Input: dimensioned drawing with shaded views. Units: mm. Origin: part minimum x, y, z. A direction names the side the tool comes from. Round coordinates to 2 decimals unless told otherwise and drop trailing zeros. Write each loop counter-clockwise with the first axis right and the second up, starting at its lowest first coordinate (ties: lowest second). Pieces come first, ordered by that corner, then holes. Notation, with made-up numbers: (5, 71.5) - (45, 71.5) arc R29 ccw to (45, 103.5) - close; hole circle Ø2 at (85.5, -10.75). An arc over 180 degrees is marked (long way). Use one line per item in the form item = value.
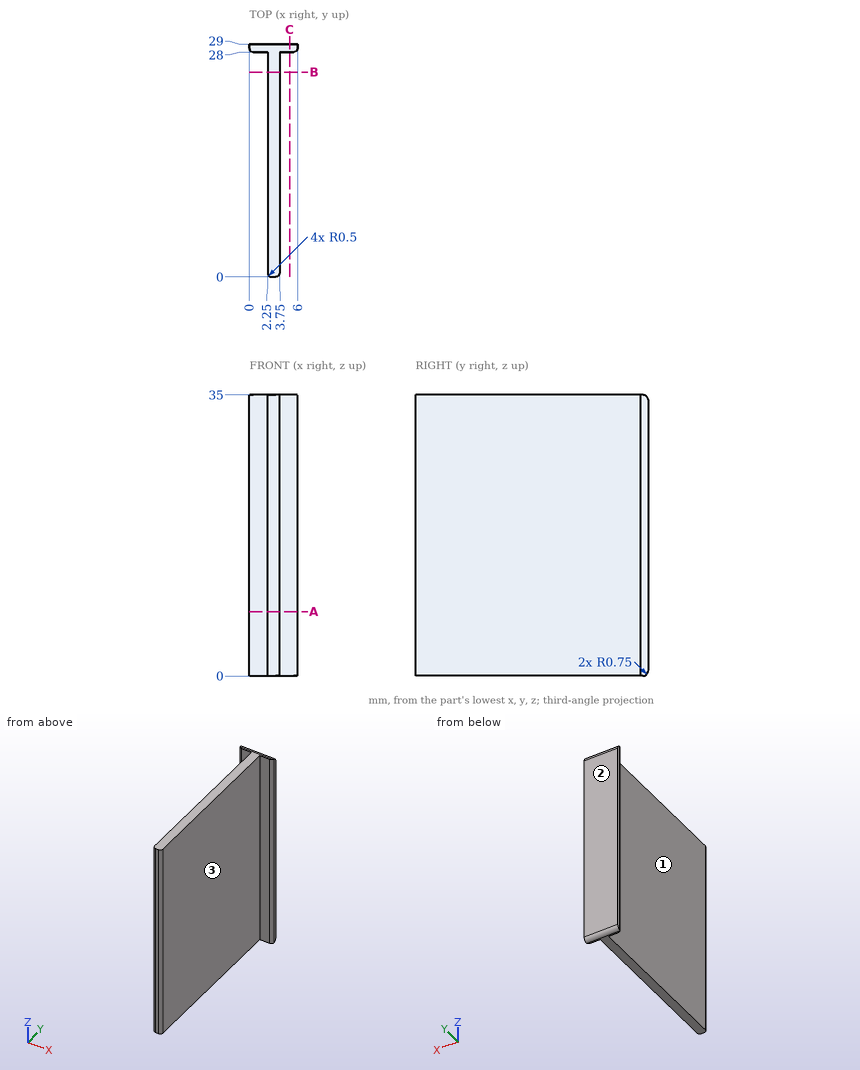
(1) Cut plane C-C on x = 5. Output: boundary loops of the cut face in (y, z), then the cut area to 3 significant figures.
Derived:
outline = (28, 0) - (28.25, 0) arc R0.75 ccw to (29, 0.75) - (29, 34.25) arc R0.75 ccw to (28.25, 35) - (28, 35) - close
area = 34.8 mm^2
(2) First-contact query: pin 1 Ø1.5 at (y, z) = (25.5, 29) entering from -X; pin 2 Ø3 at (x, z) = (1, 26) entering from -Y; pin 3 Ø4 at (y, z) = (11, 6.5) entering from +X. Flat tips, straight axial feed; report the tip coordinate or a pass-through.
Derived:
pin_1 = 2.25
pin_2 = 0.07
pin_3 = 3.75
(3) Access query for the marked faces 1, 2 and 3. Directions: +Z, -Z, +X, -X, +Y, -Y. A direction counts if a zero-diameter tool reaches every point of the face in a straight line with its end or side. Return the directions, or none.
Derived:
face_1 = +Z, -Z, -X, -Y
face_2 = +Z, -Z, +X, -X, +Y
face_3 = +Z, -Z, +X, -Y
(4) Cut plane B-B on y = 25.5. Output: boundary loops of the cut face in (x, z), then the cut area to 3 significant figures.
Derived:
outline = (2.25, 0) - (3.75, 0) - (3.75, 35) - (2.25, 35) - close
area = 52.5 mm^2
(5) Material intervals for L1, parallel to X at y = 18.25, z = 8; L2, parallel to Y at x = 4, z = 21; L3, parallel to Y at x = 2.5, z = 27.5, sorted ascending.
Derived:
L1 = 2.25 to 3.75
L2 = 28 to 29
L3 = 0.07 to 29
(6) Cut plane A-A on z = 8. Output: boundary loops of the cut face in (x, y).
Derived:
outline = (0, 28.5) arc R0.5 ccw to (0.5, 28) - (2.25, 28) - (2.25, 0.5) arc R0.5 ccw to (2.75, 0) - (3.25, 0) arc R0.5 ccw to (3.75, 0.5) - (3.75, 28) - (5.5, 28) arc R0.5 ccw to (6, 28.5) - (6, 29) - (0, 29) - close
